Read the model definition and answer for the solid it produces. Units are mm, in the model's axes. A direction names the side the tool comes from. Give positions to 0.01 mm unless a question says otherwise; leave off trailing zeros. Order: outer loops, then holes, each group sorted by start corner. A loop starts at its lowest first (then second) coordinate and runs counter-clockwise, first axis right, second up. Notation, with made-up numbers: (-3.75, 11.25) - (27.25, 11.25) arc R27 ccw to (27.25, 50.25) - close; hole circle Ø6 at (-13.5, 35). An arc over 180 degrees is marked (long way). Write each question's results on one line, items separated by ' | '. Start each with the question number.
Q1. Find section D-D on x = 31.5. Give the vertices of the cut face in (y, z), and give its area (3 significant figures).
Q2. A tool of negligible diameter and unlimited length cuts with its end or side. For faces 1 (the face through (45, 75, 4)), 2 (the face through (26, 60, 4)), 3 (the face through (30.4, 74.8, 8)), 4 (the face through (17, 68, 45)), 5 (the face through (3.944, 45.21, 36.053)), from which of +Z, -Z, +X, -X, +Y, -Y can it reach the whole face along a straight path? Write none if from no direction.
Q3. Find the intervals of material crossed by line 1 along Z through (x, y) = (36, 69.5); line 2 along Y through (x, z) = (22, 5); line 3 along X through (y, z) = (64.5, 29), in increasing order. Write a range as from..to.
Q4. Find section A-A on x = 22.5. Give the vertices of the cut face in (y, z), and give its area (3 significant figures).
Q5. For a pull along Z with two mould halves and no side action, classify faces 6 (the face through (30.4, 74.8, 37)), 7 (the face through (8, 34, 23)), 8 (the face through (7, 90, 22)), 9 (the face through (17, 64, 0)) as +Z half, -Z half, draft (parallel to the pull), parting line (faces both ways), or undercut.
Q6. Find section C-C on z = 4. Give the vertices of the cut face in (x, y).
Q7. Flat-ended cylindrical pins translate along their axes: P1, Ø4, axis at y = 9.5, z = 7.5, coming from the +X side; P2, Ø9, axis at x = 22.5, y = 75, coming from the +Z side; P3, Ø9, axis at x = 18.5, z = 4.5, coming from the -Y side. Find the tip coordinate at first contact, or state that the pin passes through.
Q8. Find section B-B on y = 75. Give the vertices of the cut face in (x, z), and give its area (3 significant figures).
from build123d import *

# Parameters (mm, degrees)
F1_DEPTH = 8
F2_W     = 30
F2_H     = 8
F3_DEPTH = 37
F4_R     = 7.5
F5_DEPTH = 45.001


with BuildPart() as f1:
    # F0 (on Right) → F1 (new body)
    with BuildSketch(Plane.YZ):
        Polygon((0, 45), (0, 0), (90, 0), (90, 45), (60, 45), (30, 26.851851), (30, 45), align=None)
    extrude(amount=F1_DEPTH)

    # F2 (on face) → F3 (join)
    with BuildSketch(Plane.YZ.offset(8)):
        with Locations((75, 41)):
            Rectangle(F2_W, F2_H)
        with Locations((75, 4)):
            Rectangle(F2_W, F2_H)
    extrude(amount=F3_DEPTH)

    # F4 (on face) → F5 (cut, through all)
    with BuildSketch(Plane.XY.offset(45)):
        with Locations((22.5, 75)):
            Circle(F4_R)
    extrude(amount=-F5_DEPTH, mode=Mode.SUBTRACT)


solid = f1.part
Working result:
1) outline: (60, 0) - (90, 0) - (90, 8) - (60, 8) - close; (60, 37) - (90, 37) - (90, 45) - (60, 45) - close | area: 480 mm²
2) face 1: +Z, -Z, +X, +Y, -Y | face 2: +Z, -Z, +X, -Y | face 3: +X, +Y, -Y | face 4: +Z, +X, -X, +Y, -Y | face 5: +Z, +X, -X
3) line 1: 0..8, 37..45 | line 2: 60..67.52, 82.48..90 | line 3: 0..8
4) outline: (60, 0) - (67.5, 0) - (67.5, 8) - (60, 8) - close; (60, 37) - (67.5, 37) - (67.5, 45) - (60, 45) - close; (82.5, 0) - (90, 0) - (90, 8) - (82.5, 8) - close; (82.5, 37) - (90, 37) - (90, 45) - (82.5, 45) - close | area: 240 mm²
5) face 6: undercut | face 7: undercut | face 8: draft | face 9: -Z half
6) outline: (0, 0) - (8, 0) - (8, 60) - (45, 60) - (45, 90) - (0, 90) - close; hole circle Ø15 at (22.5, 75)
7) P1: x = 8 | P2: through | P3: y = 60
8) outline: (0, 0) - (15, 0) - (15, 8) - (8, 8) - (8, 37) - (15, 37) - (15, 45) - (0, 45) - close; (30, 0) - (45, 0) - (45, 8) - (30, 8) - close; (30, 37) - (45, 37) - (45, 45) - (30, 45) - close | area: 712 mm²
